```python
from build123d import *

# Parameters (mm, degrees)
SKETCH1_R           = 4.75
BOSS_EXTRUDE1_DEPTH = 2.5
FILLET1_R           = 5
CUT_EXTRUDE1_REACH  = 92.275
SKETCH3_W           = 5
SKETCH3_H           = 10
BOSS_EXTRUDE2_DEPTH = 5


with BuildPart() as part:
    # Sketch1 → Boss-Extrude1 (new, symmetric)
    with BuildSketch(Plane.YZ):
        with BuildLine():
            Line((-15.757717512, 0), (-5, 0))
            Line((-5, 0), (-5, -5))
            Line((-5, -5), (5, -5))
            Line((5, -5), (5, 0))
            Line((5, 0), (14.242282488, 0))
            Line((14.242282488, 0), (12.716235334, 20.927285791))
            ThreePointArc((12.716235334, 20.927285791), (0.446501859, 32.742179409), (-12.620138577, 21.815103933))
            Line((-12.620138577, 21.815103933), (-32.620138577, 21.815103933))
            Line((-32.620138577, 21.815103933), (-44.997717512, 50))
            Line((-44.997717512, 50), (-59.997717512, 50))
            Line((-59.997717512, 50), (-74.997717512, 30))
            Line((-74.997717512, 30), (-74.997717512, 0))
            Line((-74.997717512, 0), (-15.757717512, 0))
        make_face()
        with Locations(Location((0, 20, 0), (0, 0, 270))):
            Circle(SKETCH1_R, mode=Mode.SUBTRACT)
    extrude(amount=BOSS_EXTRUDE1_DEPTH, both=True)

    # Fillet1
    fillet1_edges = [part.edges().sort_by_distance(p)[0] for p in [
        (0, -74.997717512, 30),
        (0, -59.997717512, 50),
        (0, -44.997717512, 50),
        (0, -32.620138577, 21.815103933),
        (0, -12.620138577, 21.815103933),
    ]]
    fillet(fillet1_edges, radius=FILLET1_R)

    # Sketch2 → Cut-Extrude1 (cut, up to next)
    with BuildSketch(Plane.YZ.offset(2.5), mode=Mode.PRIVATE) as cut_extrude1_sk1:
        Polygon((-50.466178577, 27.886908691), (-59.529256447, 32.113091309), (-57.416165138, 36.644630244), (-48.353087268, 32.418447626), align=None)
    cut_extrude1_tool1 = extrude(cut_extrude1_sk1.sketch, amount=-CUT_EXTRUDE1_REACH, mode=Mode.PRIVATE) & part.part
    add(cut_extrude1_tool1.solids().sort_by_distance((2.5, -53.941172, 32.265769))[0], mode=Mode.SUBTRACT)

    # Sketch3 → Boss-Extrude2 (add)
    with BuildSketch(Plane(origin=(0, 0, 0), x_dir=(1, 0, 0), z_dir=(0, 0, -1))):
        with Locations((0, 50)):
            Rectangle(SKETCH3_W, SKETCH3_H)
    extrude(amount=BOSS_EXTRUDE2_DEPTH)


solid = part.part
```
Could you check a few things on this model? Use its own coordinates, in mm. A direction names the side the tool comes from. Round coordinates to 2 decimals unless told otherwise and drop trailing zeros. Loops run counter-clockwise (first coordinate to the right, second up) from the corner with the lowest first, then second, coordinate; pieces in that order, holes last. Notation, with made-up numbers: M -24.75,-35.75 L 7.25,-35.75 A25 ccw 7.25,-10.75 Z; hole C 48.5,26 d7. An arc over 180 degrees is marked long. Answer as CSV lines item,"result".
1) Imagine slicing it at C-C on z = -1. List the corners of the cut face in (x, y) for me, and give its area (3 significant figures).
From the geometry:
outline,"M -2.5,-55 L 2.5,-55 L 2.5,-45 L -2.5,-45 Z; M -2.5,-5 L 2.5,-5 L 2.5,5 L -2.5,5 Z"
area,"100 mm^2"
2) Imagine slicing it at A-A on y = 0. List the corners of the cut face in (x, z) for me.
From the geometry:
outline,"M -2.5,-5 L 2.5,-5 L 2.5,15.25 L -2.5,15.25 Z; M -2.5,24.75 L 2.5,24.75 L 2.5,32.75 L -2.5,32.75 Z"
3) For pin 1 Ø2.5 at (x, y) = (-1, -28) entering from -Z; pin 2 Ø1.5 at (x, z) = (0, -3) entering from +Y; pin 3 Ø1.5 at (x, z) = (-0.5, -3.5) entering from -Y; pin 4 Ø12.5 at (y, z) = (0, 20) entering from +X, each with a flat end and sliding along its axis, tell me the tip position at first contact or that it passes through.
From the geometry:
pin 1,"z = 0"
pin 2,"y = 5"
pin 3,"y = -55"
pin 4,"x = 2.5"
4) If I drill on probe 1 along Y at (x, z) = (-0.8, 29); probe 2 along Y at (x, z) = (-0.6, 31.5); probe 3 along Y at (x, z) = (1.9, -1), over which ranges is the centre line in solid material (lowest first)?
From the geometry:
probe 1,"-74.95 to -52.85, -49.95 to -35.78, -9.03 to 9.03"
probe 2,"-73.87 to -58.21, -48.78 to -36.87, -5.51 to 5.51"
probe 3,"-55 to -45, -5 to 5"
5) We'd pull the mould along Z, two halves only. Please class faces 1 (the cylindrical face through (0.035, 2.275, 32.545)), 2 (the flat face through (0.04, -52.95, 34.56)), 3 (the flat face through (0, -45, -2)): released by +Z, released by -Z, zero draft, split by the parting line, or undercut.
From the geometry:
face 1,"released by +Z"
face 2,"undercut"
face 3,"zero draft"
6) Imagine slicing it at D-D on y = -36.5. List the corners of the cut face in (x, z) for me, and give its area (3 significant figures).
From the geometry:
outline,"M -2.5,0 L 2.5,0 L 2.5,30.65 L -2.5,30.65 Z"
area,"153 mm^2"
7) Imagine slicing it at B-B on x = -0.2. List the corners of the cut face in (y, z) for me.
From the geometry:
outline,"M -75,0 L -55,0 L -55,-5 L -45,-5 L -45,0 L -5,0 L -5,-5 L 5,-5 L 5,0 L 14.24,0 L 12.72,20.93 A12.75 ccw -11.77,24.9 A5 cw -16.39,21.82 L -29.36,21.82 A5 cw -33.93,24.8 L -43.68,47.01 A5 ccw -48.26,50 L -57.5,50 A5 ccw -61.5,48 L -74,31.33 A5 ccw -75,28.33 Z; hole M -59.53,32.11 L -50.47,27.89 L -48.35,32.42 L -57.42,36.64 Z; hole C 0,20 d9.5"
8) Which directions (+Z, -Z, +X, -X, +Y, -Y) give clear straight access to the entire face, cutting with the end or side of a thin tool? Please do faces 4 (the cylindrical face through (-0.04, -32.12, 22.65)), 5 (the flat face through (0, -55, -2)), 6 (the flat face through (0.035, -58.488, 34.347)).
From the geometry:
face 4,"+Z, +X, -X"
face 5,"-Z, +X, -X, -Y"
face 6,"+X, -X"
